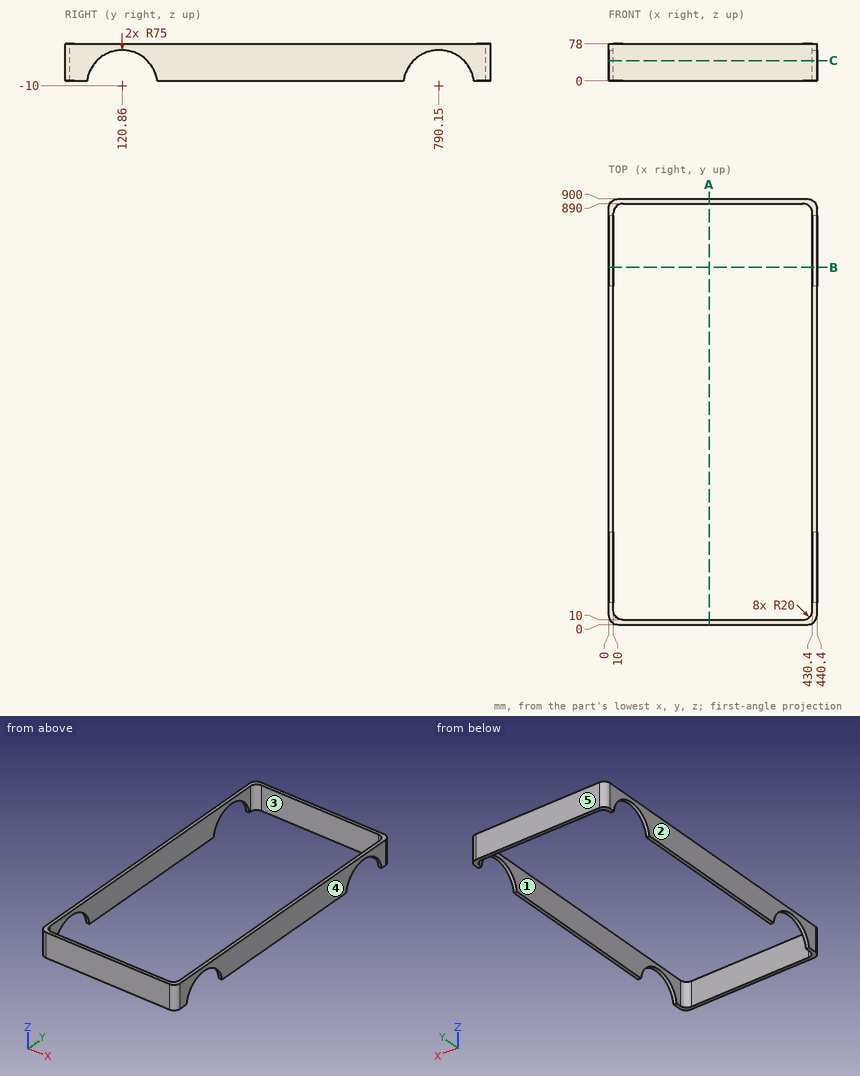
Can you work these out from the drawing? Everything is in mm from the part's minimum corner. A direction names the side the tool comes from. Give positions to 0.01 mm unless a question says otherwise; leave off trailing zeros. Loops run counter-clockwise (first coordinate to the right, second up) from the corner with the lowest first, then second, coordinate; pieces in that order, holes last. Notation, with made-up numbers: M 75.5,28 L 105.5,28 A23 cw 105.5,40 Z; hole C 14,27.5 d7. An arc over 180 degrees is marked long. Put each result on its own line as item: value. Start each with the question number.
(1) I need wall thicknesses on line 1 along Y through (x, z) = (155, 17.5); line 2 along X through (y, z) = (570.5, 69.5). Which ranges of each line are inside material? Lowest first, please. Write a range as [from, to].
(2) I want a section at A-A on x = 212.5. Please give me the cut outline in (y, z), then the cut area to 3 significant figures.
(3) For the marked faces 1 and 2, which set-ups out of +Z, -Z, +X, -X, +Y, -Y let a thin tool reach every point of the face, with its end or its side?
(4) Will this pin go through, and if not, where does the flat tip stop? pin 1 Ø10 at (y, z) = (331, 66) entering from -X.
(5) I want a section at C-C on z = 43. State how many separate pieces and enclosed holes the cut face has, then the cut area to 3 significant figures.
(6) If we mould it in two halves opening along Y, with no side actions, what happens to the marked faces 3, 4 and 5? For each: +Y half, -Y half, draft (parallel to the pull), parting line (faces both ways), or undercut.
(7) I want a section at B-B on y = 755. Please give me the cut outline in (x, z), then the cut area to 3 significant figures.
Answer block:
1. line 1: [0, 10], [890, 900]
1. line 2: [0, 10], [430.4, 440.4]
2. outline: M 0,0 L 10,0 L 10,78 L 0,78 Z; M 890,0 L 900,0 L 900,78 L 890,78 Z
2. area: 1,560 mm^2
3. face 1: +Z, -Z
3. face 2: +Z, -Z, -X, +Y, -Y
4. pin 1: x = 0
5. separate pieces: 4
5. enclosed holes: 0
5. area: 22,200 mm^2
6. face 3: undercut
6. face 4: draft
6. face 5: +Y half
7. outline: M 0,56.25 L 10,56.25 L 10,78 L 0,78 Z; M 430.4,56.25 L 440.4,56.25 L 440.4,78 L 430.4,78 Z
7. area: 435 mm^2
